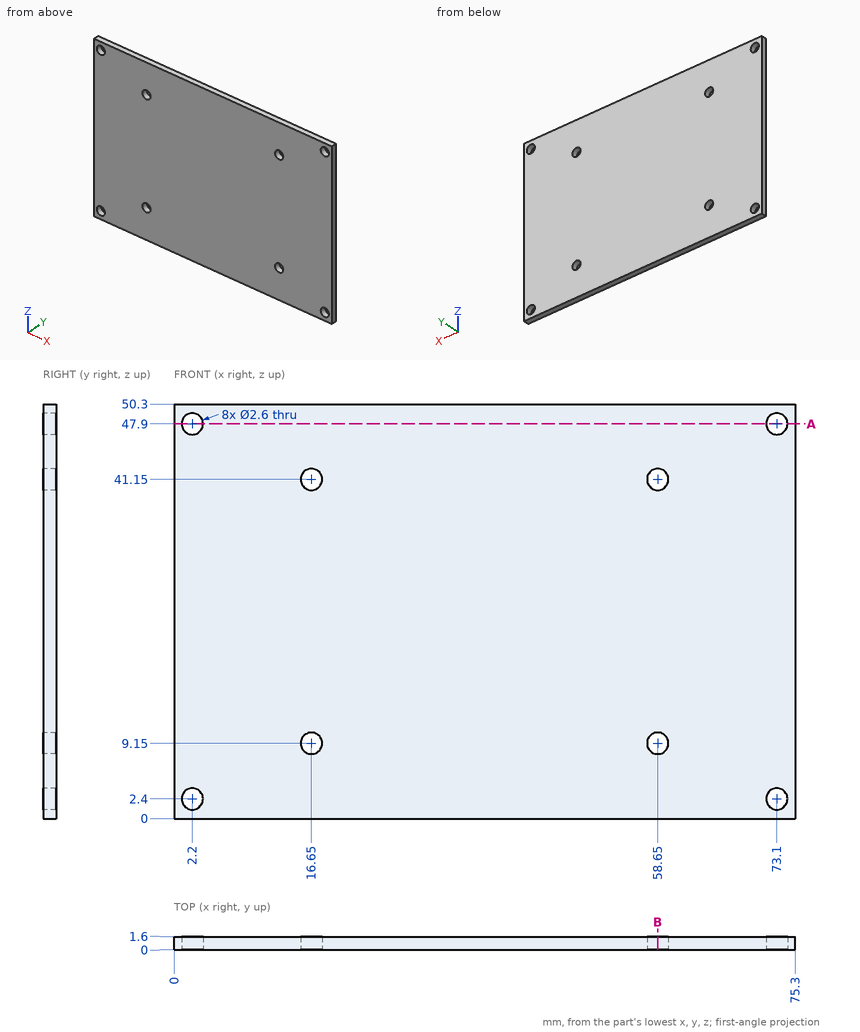
Print and shaded views of the part. All mm, measured from the part's lowest x, y and z. Coordinates: 2 decimals unless noted, no trailing zeros. Write each loop counter-clockwise with the first axis right and the second up, starting at its lowest first coordinate (ties: lowest second). Pieces come first, ordered by that corner, then holes. Notation, with made-up numbers: M 54,37 L 101,37 A29 cw 101,65 Z; hole C 38.5,83 d11. An arc over 180 degrees is marked long. Return JSON: item names as keys, results as strings.
1. Saw through at B-B, the plane x = 58.65. Write the cut outline in (y, z), then the cut area to 3 significant figures.
Determined:
{"outline": "M 0,0 L 1.6,0 L 1.6,7.85 L 0,7.85 Z; M 0,10.45 L 1.6,10.45 L 1.6,39.85 L 0,39.85 Z; M 0,42.45 L 1.6,42.45 L 1.6,50.3 L 0,50.3 Z", "area": "72.2 mm²"}
2. Flat gauge pins, fed straight in: pin 1 Ø1.6 at (x, z) = (58.65, 9.15) entering from +Y; pin 2 Ø3 at (x, z) = (16.65, 9.15) entering from +Y. Where does each tip first touch, or does it go through?
Determined:
{"pin 1": "through", "pin 2": "y = 1.6"}
3. Saw through at A-A, the plane z = 47.9. Write the cut outline in (x, y).
Determined:
{"outline": "M 0,0 L 0.9,0 L 0.9,1.6 L 0,1.6 Z; M 3.5,0 L 71.8,0 L 71.8,1.6 L 3.5,1.6 Z; M 74.4,0 L 75.3,0 L 75.3,1.6 L 74.4,1.6 Z"}
4. Probe L1, parallel to X at y = 1.1, z = 41.15; L2, parallel to Z at x = 2.2, y = 0.5; L3, parallel to Z at x = 58.65, y = 0.65. List the from-to ranges inside material, lowest first.
Determined:
{"L1": "0 to 15.35, 17.95 to 57.35, 59.95 to 75.3", "L2": "0 to 1.1, 3.7 to 46.6, 49.2 to 50.3", "L3": "0 to 7.85, 10.45 to 39.85, 42.45 to 50.3"}
